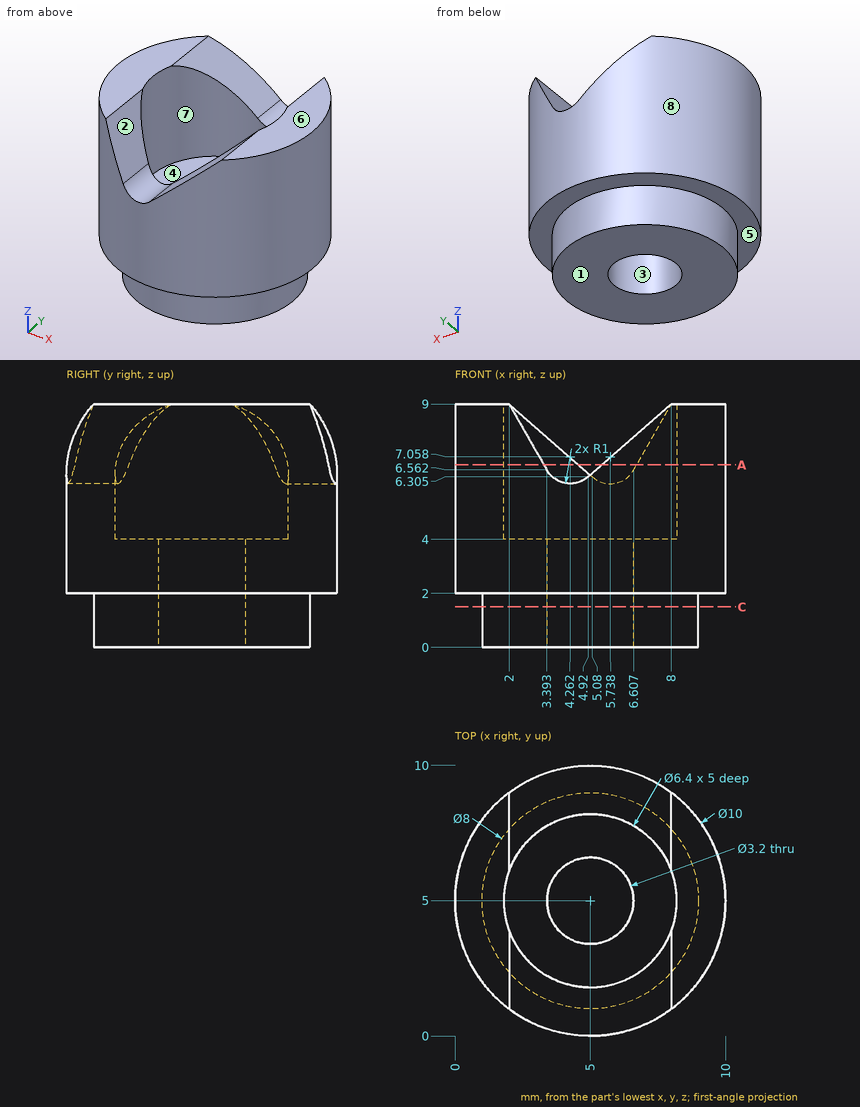
Drawing for the job (mm, zero at the part's lowest x, y, z). A direction names the side the tool comes from. Round coordinates to 2 decimals unless told otherwise and drop trailing zeros. Write each loop counter-clockwise with the first axis right and the second up, starting at its lowest first coordinate (ties: lowest second). Pieces come first, ordered by that corner, then holes. Notation, with made-up numbers: (52.25, 31) - (85.25, 31) arc R18 cw to (85.25, 61) - close; hole circle Ø10 at (-27.5, 65.5). An arc over 180 degrees is marked (long way). Return JSON: item names as keys, results as strings. Group by question number.
Item 1: Band-saw the part on A-A on z = 6.75. List the corners of the cut face in (x, y) (1 decimal).
Item 2: Flat gauge pins, fed straight in: pin 1 Ø1.5 at (y, z) = (7.5, 6) entering from +X; pin 2 Ø1 at (x, z) = (3.5, 7) entering from -Y; pin 3 Ø2 at (x, y) = (4, 1.5) entering from +Z. Where does each tip first touch, or does it go through?
Item 3: Probe probe 1 along Y at (x, z) = (5, 5.4); probe 2 along Z at (x, y) = (0.5, 6.5); probe 3 along Y at (x, z) = (8, 3). List the from-to ranges inside material, lowest first.
Item 4: 3-axis set-ups, long thin cutter, end or side, ignore diameter. For the marked faces 1, 2, 3, 4 and 5: which of +Z, -Z, +X, -X, +Y, -Y reach the whole face in a straight line?
Item 5: Mould opens along Y. For the marked faces 6, 7 and 8 say: +Y half, -Y half, draft (parallel to the pull), parting line (faces both ways), or undercut.
Item 6: Band-saw the part on C-C on z = 1.5. List the corners of the cut face in (x, y).
Resolved:
{
 "1": {"outline": "(3.3, 0.3) - (3.3, 2.3) arc R3.2 cw to (4.6, 8.2) - (4.6, 10) arc R5 ccw to start; (5.4, 0) arc R5 ccw to (6.7, 9.7) - (6.7, 7.7) arc R3.2 cw to (5.4, 1.8) - close"},
 "2": {"pin 1": "stops at x = 9.68", "pin 2": "stops at y = 0.25", "pin 3": "stops at z = 7.25"},
 "3": {"probe 1": "y = 0 to 1.8, 8.2 to 10", "probe 2": "z = 2 to 9", "probe 3": "y = 1 to 9"},
 "4": {"face 1": "-Z, +X, -X, +Y, -Y", "face 2": "+Z, -Y", "face 3": "+Z, -Z", "face 4": "+Z", "face 5": "-Z"},
 "5": {"face 6": "draft", "face 7": "undercut", "face 8": "parting line"},
 "6": {"outline": "circle Ø8 at (5, 5); hole circle Ø3.2 at (5, 5)"}
}
